Check sheet for the modelled part. Datum: model origin and axes. Units: mm. Round coordinates to 2 decimals unless told otherwise and drop trailing zeros. Order: outer loops, then holes, each group sorted by start corner. A loop starts at its lowest first (then second) coordinate and runs counter-clockwise, first axis right, second up.
```python
from build123d import *

# Parameters (mm, degrees)
SKETCH_1_W          = 78
SKETCH_1_H          = 241
EXTRUDE_1_DEPTH     = 3
EXTRUDE_2_DEPTH     = 3
SKETCH_5_W          = 3
SKETCH_5_H          = 30
SKETCH_5_H_2        = 61
CUT_EXTRUDE_3_DEPTH = 3
SKETCH_6_W          = 3
SKETCH_6_H          = 30
SKETCH_6_H_2        = 61
CUT_EXTRUDE_4_DEPTH = 3
SKETCH_7_W          = 10
SKETCH_7_H          = 30
CUT_EXTRUDE_5_DEPTH = 3
FILLET_1_R          = 10
HOLE_WIZARD_M4_1_D  = 3.3
HOLE_WIZARD_M3_2_D  = 2.5


with BuildPart() as part:
    # 草图1 → 凸台-拉伸1 (new body)
    with BuildSketch(Plane.XY):
        with Locations((37.174772521, -24.067785913)):
            Rectangle(SKETCH_1_W, SKETCH_1_H)
    extrude(amount=-EXTRUDE_1_DEPTH)

    # 草图2 → 凸台-拉伸2 (add)
    with BuildSketch(Plane.XY):
        Polygon((-1.825227479, 96.432214087), (-126.825227479, 23.432214087), (-126.825227479, -71.567785913), (-1.825227479, -144.567785913), align=None)
    extrude(amount=-EXTRUDE_2_DEPTH)

    # 草图5 → 切除-拉伸3 (cut)
    with BuildSketch(Plane.XY):
        with Locations((74.674772521, 61.432214087)):
            Rectangle(SKETCH_5_W, SKETCH_5_H)
        with Locations((74.674772521, -109.567785913)):
            Rectangle(SKETCH_5_W, SKETCH_5_H)
        with Locations((74.674772521, -24.067785913)):
            Rectangle(SKETCH_5_W, SKETCH_5_H_2)
    extrude(amount=-CUT_EXTRUDE_3_DEPTH, mode=Mode.SUBTRACT)

    # 草图6 → 切除-拉伸4 (cut)
    with BuildSketch(Plane(origin=(0, 0, -3), x_dir=(-1, 0, 0), z_dir=(0, 0, -1))):
        with Locations((-2.674772521, 61.432214087)):
            Rectangle(SKETCH_6_W, SKETCH_6_H)
        with Locations((-2.674772521, -24.067785913)):
            Rectangle(SKETCH_6_W, SKETCH_6_H_2)
        with Locations((-2.674772521, -109.567785913)):
            Rectangle(SKETCH_6_W, SKETCH_6_H)
    extrude(amount=-CUT_EXTRUDE_4_DEPTH, mode=Mode.SUBTRACT)

    # 草图7 → 切除-拉伸5 (cut)
    with BuildSketch(Plane.XY):
        with Locations((12.174772521, -88.567785913)):
            Rectangle(SKETCH_7_W, SKETCH_7_H)
    extrude(amount=-CUT_EXTRUDE_5_DEPTH, mode=Mode.SUBTRACT)

    # 圆角1
    fillet_1_edges = [part.edges().sort_by_distance(p)[0] for p in [
        (-126.825227479, -71.567785913, -1.5),
        (-126.825227479, 23.432214087, -1.5),
        (-1.825227479, 96.432214087, -1.5),
        (-1.825227479, -144.567785913, -1.5),
        (76.174772521, -144.567785913, -1.5),
        (76.174772521, 96.432214087, -1.5),
    ]]
    fillet(fillet_1_edges, radius=FILLET_1_R)

    # M4 螺纹孔的螺纹孔钻头1 (through all)
    with Locations(Plane(origin=(-111.825227479, 13.432214087, -3), x_dir=(-1, 0, 0), z_dir=(0, 0, -1))):
        with Locations((0, 0), (0, -75), (-75, -75), (-75, 0)):
            Hole(HOLE_WIZARD_M4_1_D / 2)

    # M3 螺纹孔的螺纹孔钻头2 (through all)
    with Locations(Plane(origin=(63.174772521, -131.567785913, -3), x_dir=(-1, 0, 0), z_dir=(0, 0, -1))):
        with Locations((0, 0), (49, 0), (0, 215), (49, 215)):
            Hole(HOLE_WIZARD_M3_2_D / 2)


solid = part.part
```
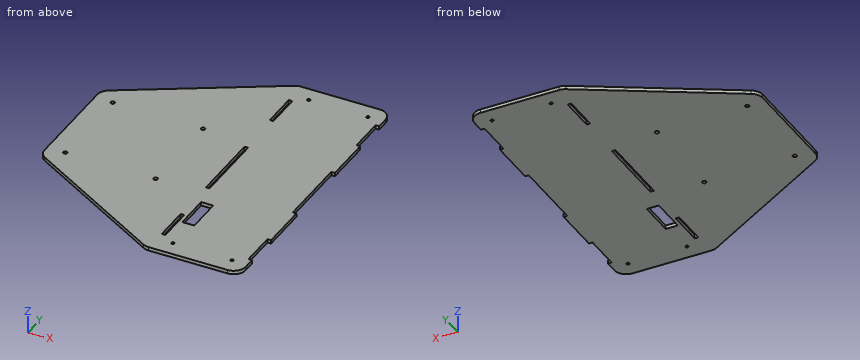
Item 1: Go/stop test with a flat-tipped pin: P1, Ø1.5, axis at y = 68.5, z = -2, coming from the +X side. Record where the tip stops, or that it passes through.
Answer:
P1: stops at x = 73.17
Item 2: Sectioned sample at C-C (x = -10). Record the cut outline in (y, z).
Answer:
outline: (-139.79, -3) - (91.66, -3) - (91.66, 0) - (-139.79, 0) - close
Item 3: Scan lines: line 1 along X through (y, z) = (-74.5, -1.65); line 2 along X through (y, z) = (-13.5, -2.1); line 3 along Y through (x, z) = (17, -0.9). Record each from-to range of solid material in increasing order.
Answer:
line 1: x = -121.8 to 7.17, 17.17 to 76.17
line 2: x = -126.83 to 1.17, 4.17 to 73.17
line 3: y = -144.57 to -103.57, -73.57 to 96.43
Item 4: Sectioned sample at A-A (y = -10). Record the cut outline in (x, z), and give its area (3 significant figures).
Answer:
outline: (-126.83, -3) - (1.17, -3) - (1.17, 0) - (-126.83, 0) - close; (4.17, -3) - (73.17, -3) - (73.17, 0) - (4.17, 0) - close
area: 591 mm2
Item 5: Sectioned sample at B-B (y = -81.5). Record the cut outline in (x, z).
Answer:
outline: (-109.82, -3) - (7.17, -3) - (7.17, 0) - (-109.82, 0) - close; (17.17, -3) - (76.17, -3) - (76.17, 0) - (17.17, 0) - close
Item 6: Sectioned sample at D-D (z = -0.7). State how many separate pieces and enclosed holes the cut face has, and give its area (3 significant figures).
Answer:
separate pieces: 1
enclosed holes: 12
area: 38,700 mm2
